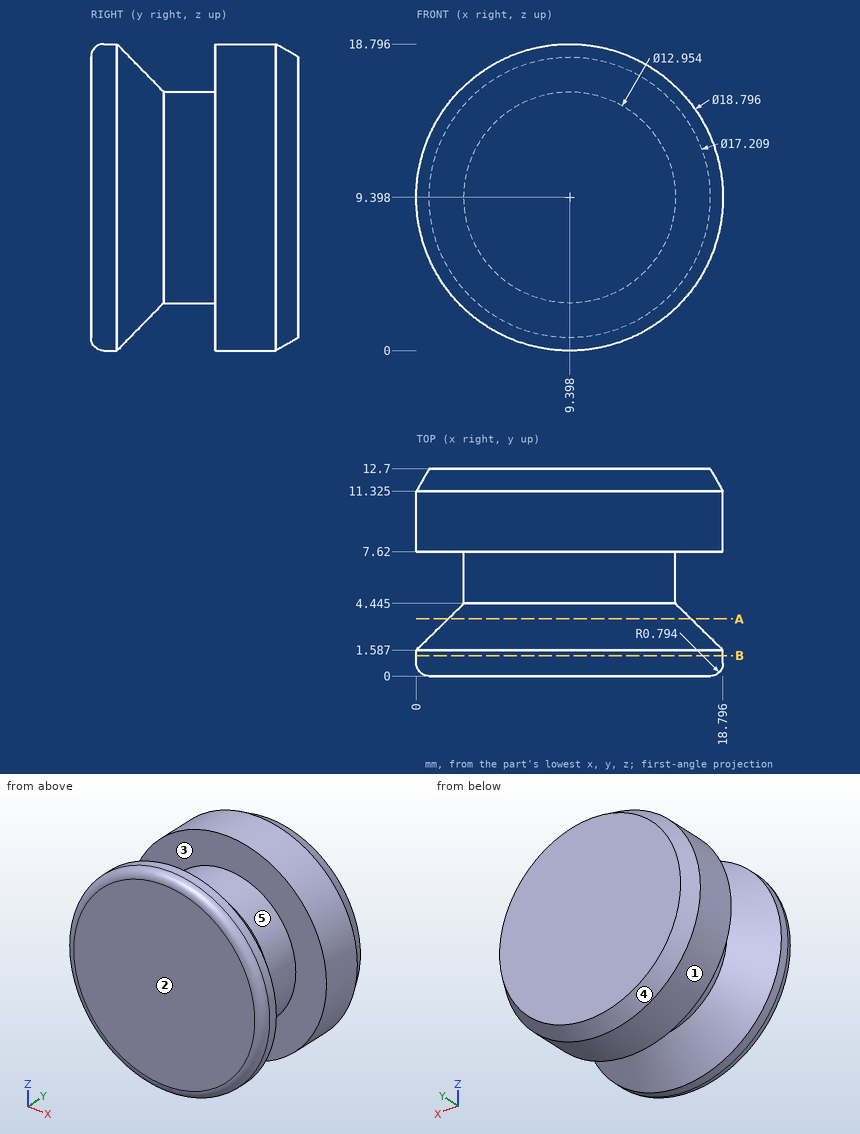
Can you work these out from the drawing? Everything is in mm from the part's minimum corner. A direction names the side the tool comes from. Round coordinates to 2 decimals unless told otherwise and drop trailing zeros. Loops run counter-clockwise (first coordinate to the right, second up) from the corner with the lowest first, then second, coordinate; pieces in that order, holes last. Notation, with made-up numbers: (68.25, -35.75) - (88.25, -35.75) arc R27 cw to (88.25, -2.75) - close; hole circle Ø5 at (12.25, 56). An arc over 180 degrees is marked (long way). Write item = value, one per line. Start each with the question number.
(1) For P1, Ø1, axis at x = 9, y = 6, coming from the +Z side (1 decimal); P2, Ø1, axis at y = 2, z = 10.5, coming from the +X side; P3, Ø5, axis at x = 2.5, y = 4, coming from the +Z side, each with a flat end and sliding along its axis, tell me the tip position at first contact or that it passes through.
(2) If I drill on probe 1 along Y at (x, z) = (12.25, 17.5); probe 2 along Y at (x, z) = (15.5, 16) (1 decimal); probe 3 along X at (y, z) = (10.75, 9.25) (1 decimal), over which ranges is the centre line in solid material (lowest first)? Write a range as [from, to].
(3) If we mould it in two halves opening along Y, with no side actions, what happens to the marked faces 1, 2 and 3? For each: released by +Y, released by -Y, zero draft, split by the parting line, or undercut.
(4) For the marked faces 4 and 5, which set-ups out of +Z, -Z, +X, -X, +Y, -Y let a thin tool reach every point of the face, with its end or its side?
(5) If we section it at B-B (y = 1.25): Please give me the cut outline in (x, z) (1 decimal).
(6) If we section it at A-A (y = 3.5): Please give me the cut outline in (x, z) (1 decimal), and give its area (3 significant figures).
Ans:
q1.P1 = 15.9
q1.P2 = 18.76
q1.P3 = 16.59
q2.probe_1 = [0, 2.38], [7.62, 12.7]
q2.probe_2 = [0.1, 2], [7.6, 12]
q2.probe_3 = [0, 18.8]
q3.face_1 = zero draft
q3.face_2 = released by -Y
q3.face_3 = undercut
q4.face_4 = +Y
q4.face_5 = none
q5.outline = circle Ø18.8 at (9.4, 9.4)
q6.outline = circle Ø14.9 at (9.4, 9.4)
q6.area = 174 mm²
